from build123d import *

# Parameters (mm, degrees)
PAD_DEPTH = 29.21


with BuildPart() as part:
    # Sketch → Pad (new body)
    with BuildSketch(Plane.XY):
        with BuildLine():
            ThreePointArc((1.5875, -11.83454), (0, 11.94054), (-1.5875, -11.83454))
            Line((-1.5875, -11.83454), (-1.5875, -24.589348))
            ThreePointArc((-16.504081, 18.296763), (-23.272966, -8.094767), (-1.5875, -24.589348))
            Line((-16.504081, 18.296763), (16.504081, 18.296763))
            ThreePointArc((1.5875, -24.589348), (23.272966, -8.094767), (16.504081, 18.296763))
            Line((1.5875, -11.83454), (1.5875, -24.589348))
        make_face()
    extrude(amount=PAD_DEPTH)


solid = part.part
Model file for the job. Use its own axes, mm. A direction names the side the tool comes from. Give positions to 0.01 mm unless a question says otherwise; leave off trailing zeros. Order: outer loops, then holes, each group sorted by start corner. A loop starts at its lowest first (then second) coordinate and runs counter-clockwise, first axis right, second up. Notation, with made-up numbers: (23, 3) - (60, 3) arc R8 ccw to (60, 9) - close; hole circle Ø2 at (80.5, 49). An arc over 180 degrees is marked (long way). Return JSON: item names as keys, results as strings.
1) 3-axis set-ups, long thin cutter, end or side, ignore diameter. For faces 1 (the flat face through (-11, -8, 29.21)), 2 (the flat face through (1.588, -18, 14)): which of +Z, -Z, +X, -X, +Y, -Y reach the whole face in a straight line?
Geometry says:
{"face 1": "+Z, +X, -X, +Y, -Y", "face 2": "+Z, -Z, -Y"}
2) Flat gauge pins, fed straight in: P1, Ø4, axis at x = 13.5, z = 13, coming from the -Y side; P2, Ø8, axis at x = -0.5, z = 21, coming from the -Y side; P3, Ø3, axis at y = -10, z = 18.5, coming from the -X side. Where does each tip first touch, or does it go through?
Geometry says:
{"P1": "y = -21.79", "P2": "y = -24.59", "P3": "x = -23.13"}
3) Pull direction X, two halves, no side cores. Call faces 3 (the flat face through (-1.588, -18, 14)), 4 (the cylindrical face through (23.137, -8.475, 14.401)), 5 (the flat face through (-11, -8, 0)): pulls with the +X half, pulls with the -X half, needs draft (parallel to the pull), parting line crosses it, or undercut.
Geometry says:
{"face 3": "undercut", "face 4": "pulls with the +X half", "face 5": "needs draft"}
4) Cut at C-C, the plane z = 11.25. Give the cut face in (x, y).
Geometry says:
{"outline": "(-16.5, 18.3) arc R24.64 ccw to (-1.59, -24.59) - (-1.59, -11.83) arc R11.94 cw (long way) to (1.59, -11.83) - (1.59, -24.59) arc R24.64 ccw to (16.5, 18.3) - close"}
5) Probe line 1 (X direction, y = 0, z = 21.5); line 2 (Y direction, x = 9, z = 15); line 3 (X direction, y = -18.5, z = 8). List the from-to ranges inside material, lowest first. Write a range as from..to.
Geometry says:
{"line 1": "-24.64..-11.94, 11.94..24.64", "line 2": "-22.94..-7.85, 7.85..18.3", "line 3": "-16.28..-1.59, 1.59..16.28"}
6) Cut at D-D, the plane x = -21. Give the cut face in (y, z), plus the area to 3 significant figures.
Geometry says:
{"outline": "(-12.89, 0) - (12.89, 0) - (12.89, 29.21) - (-12.89, 29.21) - close", "area": "753 mm²"}
7) Cut at A-A, the plane y = 0. Give the cut face in (x, z), plus the area to 3 significant figures.
Geometry says:
{"outline": "(-24.64, 0) - (-11.94, 0) - (-11.94, 29.21) - (-24.64, 29.21) - close; (11.94, 0) - (24.64, 0) - (24.64, 29.21) - (11.94, 29.21) - close", "area": "742 mm²"}
8) Cut at B-B, the plane x = -4.5. Give the cut face in (y, z), plus the area to 3 significant figures.
Geometry says:
{"outline": "(-24.23, 0) - (-11.06, 0) - (-11.06, 29.21) - (-24.23, 29.21) - close; (11.06, 0) - (18.3, 0) - (18.3, 29.21) - (11.06, 29.21) - close", "area": "596 mm²"}
